Could you check a few things on this model? Use its own coordinates, in mm. Face numbers are marked on the shaded views. A direction names the side the tool comes from. Give positions to 0.01 mm unless a question says otherwise; leave off trailing zeros. Loops run counter-clockwise (first coordinate to the right, second up) from the corner with the lowest first, then second, coordinate; pieces in that order, holes last. Notation, with made-up numbers: (26.25, -37.5) - (83.25, -37.5) arc R18 ccw to (83.25, -17.5) - close; hole circle Ø10 at (24.5, 34.25). An arc over 180 degrees is marked (long way). Write each question's results on one line, items separated by ' | '. Start each with the question number.
(1) Suppose I cut it at D-D (z = 8.5). Please give me the cut outline in (x, y).
(2) I need wall thicknesses on line 1 (Y direction, x = 8.5, z = -1.6); line 2 (Z direction, x = 2, y = 1); line 3 (Z direction, x = -5.5, y = 1.5). Which ranges of each line are inside material? Lowest first, please.
(3) For pin 1 (1.2 mm diameter, centred on x = -20, y = 0, fed in from +Z); pin 2 (4.5 mm diameter, centred on x = 8.5, y = 0.5, fed in from -Z); pin 3 (1 mm diameter, centred on x = -15.5, y = -3.5, fed in from +Z); pin 4 (1.3 mm diameter, centred on x = 9, y = -1, fed in from +Z), each with a flat end and sliding along its axis, tell me the tip position at first contact or that it passes through.
(4) Suppose I cut it at A-A (x = -20). Please give me the cut outline in (y, z), and give its area (3 significant figures).
(5) Suppose I cut it at C-C (y = 4). Please give me the cut outline in (x, z).
(6) On a 3-axis mill with a long thin cutter (end or side, diameter ignored), from which of +Z, -Z, +X, -X, +Y, -Y can I reach the whole of each face in a straight line? I mean the marked faces 1, 2, 3, 4 and 5. Say none if no direction works.
(7) Suppose I cut it at B-B (x = -6). Please give me the cut outline in (y, z), and give its area (3 significant figures).
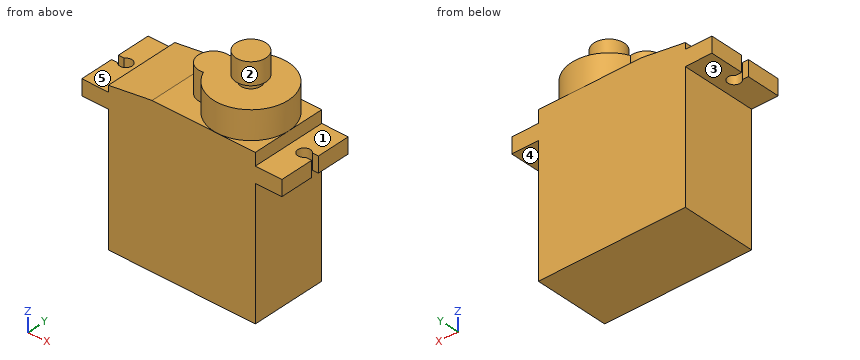
from build123d import *

# Parameters (mm, degrees)
SKETCH1_R           = 6
BOSS_EXTRUDE1_DEPTH = 6.5
SKETCH2_W           = 23.5
SKETCH2_H           = 12
BOSS_EXTRUDE2_DEPTH = 2
BOSS_EXTRUDE3_DEPTH = 2.5
SKETCH4_W           = 23.5
SKETCH4_H           = 12
BOSS_EXTRUDE4_DEPTH = 20.5
BOSS_EXTRUDE5_DEPTH = 4.5
SKETCH6_R           = 1.6
BOSS_EXTRUDE6_DEPTH = 1
SKETCH7_R           = 2.4
BOSS_EXTRUDE7_DEPTH = 3.5
CHAMFER1_SIZE       = 1
CHAMFER1_SIZE2      = 7


with BuildPart() as part:
    # Sketch1 → Boss-Extrude1 (new body)
    with BuildSketch(Plane.XY):
        with Locations(Location((0, 0, 0), (0, 0, 180))):
            Circle(SKETCH1_R)
    extrude(amount=BOSS_EXTRUDE1_DEPTH)

    # Sketch2 → Boss-Extrude2 (add)
    with BuildSketch(Plane.XY):
        with Locations((-5.75, 0)):
            Rectangle(SKETCH2_W, SKETCH2_H)
    extrude(amount=BOSS_EXTRUDE2_DEPTH)

    # Sketch3 → Boss-Extrude3 (add)
    with BuildSketch(Plane.XY):
        with BuildLine():
            Line((10.25, 6), (-21.75, 6))
            Line((-21.75, 6), (-21.75, 0.6))
            Line((-21.75, 0.6), (-20.8, 0.6))
            ThreePointArc((-20.8, 0.6), (-19, 0), (-20.8, -0.6))
            Line((-20.8, -0.6), (-21.75, -0.6))
            Line((-21.75, -0.6), (-21.75, -6))
            Line((-21.75, -6), (10.25, -6))
            Line((10.25, -6), (10.25, -0.6))
            Line((10.25, -0.6), (9.3, -0.6))
            ThreePointArc((9.3, -0.6), (7.5, 0), (9.3, 0.6))
            Line((9.3, 0.6), (10.25, 0.6))
            Line((10.25, 0.6), (10.25, 6))
        make_face()
    extrude(amount=-BOSS_EXTRUDE3_DEPTH)

    # Sketch4 → Boss-Extrude4 (add)
    with BuildSketch(Plane(origin=(0, 0, -2.5), x_dir=(-1, 0, 0), z_dir=(0, 0, -1))):
        with Locations((5.75, 0)):
            Rectangle(SKETCH4_W, SKETCH4_H)
    extrude(amount=BOSS_EXTRUDE4_DEPTH)

    # Sketch5 → Boss-Extrude5 (add)
    with BuildSketch(Plane.XY.offset(2)):
        with BuildLine():
            ThreePointArc((-5.52, -2.351510153), (-6, 0), (-5.52, 2.351510153))
            ThreePointArc((-5.52, 2.351510153), (-8.4, 0), (-5.52, -2.351510153))
        make_face()
    extrude(amount=BOSS_EXTRUDE5_DEPTH)

    # Sketch6 → Boss-Extrude6 (add)
    with BuildSketch(Plane.XY.offset(6.5)):
        Circle(SKETCH6_R)
    extrude(amount=BOSS_EXTRUDE6_DEPTH)

    # Sketch7 → Boss-Extrude7 (add)
    with BuildSketch(Plane.XY.offset(7.5)):
        Circle(SKETCH7_R)
    extrude(amount=BOSS_EXTRUDE7_DEPTH)

    # Chamfer1
    chamfer1_edges = [part.edges().sort_by_distance(p)[0] for p in [
        (-17.5, 0, 2),
    ]]
    chamfer1_side = [part.faces().sort_by_distance(p)[0] for p in [
        (-17.5, 0, 1),
    ]]
    chamfer(chamfer1_edges, length=CHAMFER1_SIZE, length2=CHAMFER1_SIZE2, reference=chamfer1_side[0])


solid = part.part
Output values:
1) outline: circle Ø4.8 at (0, 0)
2) line 1: -6 to -1, 1 to 6 | line 2: -23 to 6.5, 7.5 to 11 | line 3: -23 to 6.5
3) pin 1: through | pin 2: z = -2.5 | pin 3: z = 1.36 | pin 4: z = 0
4) outline: (-6, -2.5) - (-1, -2.5) - (-1, 0) - (-6, 0) - close; (1, -2.5) - (6, -2.5) - (6, 0) - (1, 0) - close | area: 25.0 mm2
5) outline: (-21.75, -2.5) - (-17.5, -2.5) - (-17.5, -23) - (6, -23) - (6, -2.5) - (10.25, -2.5) - (10.25, 0) - (6, 0) - (6, 2) - (4.47, 2) - (4.47, 6.5) - (-4.47, 6.5) - (-4.47, 2) - (-10.5, 2) - (-17.5, 1) - (-17.5, 0) - (-21.75, 0) - close
6) face 1: +Z, +X, +Y, -Y | face 2: +Z | face 3: -Z, -X, +Y, -Y | face 4: -Z, +X, +Y, -Y | face 5: +Z, -X, +Y, -Y
7) outline: (-6, -23) - (6, -23) - (6, 2) - (2.4, 2) - (2.4, 6.5) - (-2.4, 6.5) - (-2.4, 2) - (-6, 2) - close | area: 322 mm2
